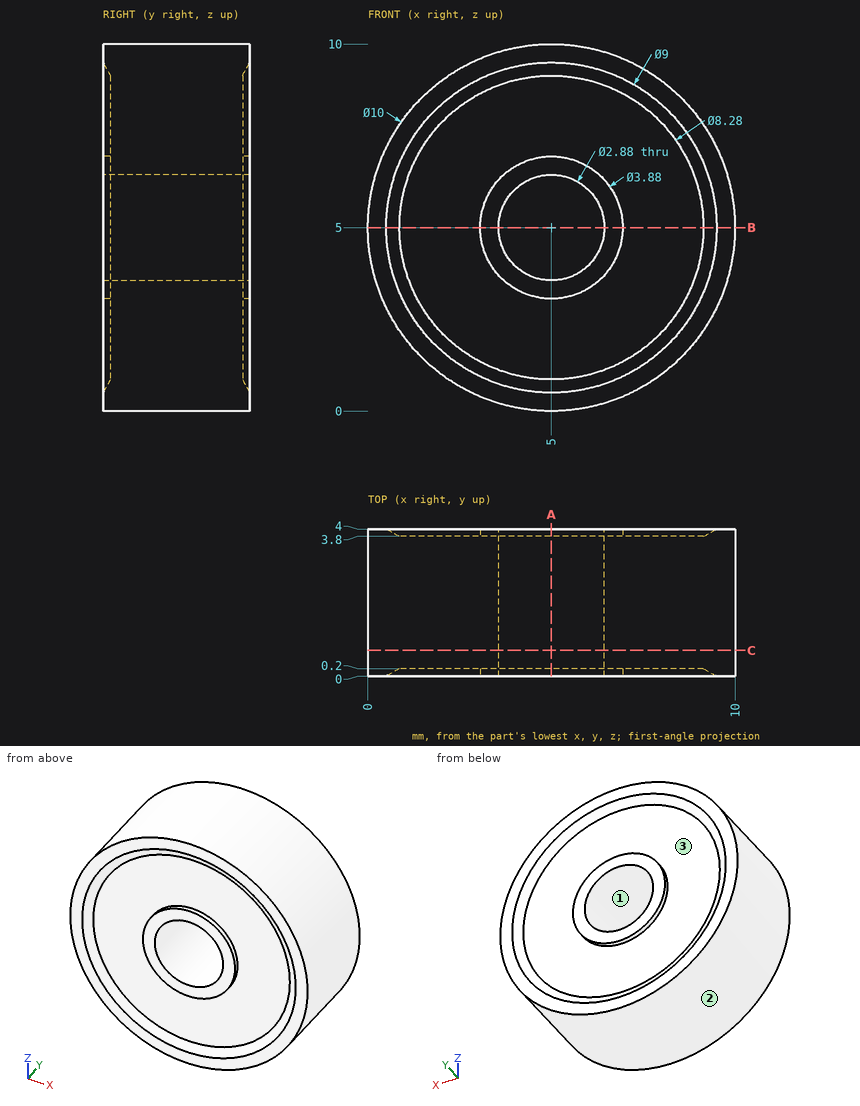
Study the drawing (mm; zero at the part's minimum x, y, z) and answer. Give positions to 0.01 mm unless a question says otherwise; leave off trailing zeros. Write each loop counter-clockwise with the first axis right and the second up, starting at its lowest first coordinate (ties: lowest second). Pieces come first, ordered by that corner, then holes.
Item 1: Flat-ended cylindrical pins translate along their axes: P1, Ø1.7, axis at x = 5, z = 5, coming from the +Y side; P2, Ø1, axis at y = 1.5, z = 7.5, coming from the +X side; P3, Ø1, axis at x = 1.5, z = 3.5, coming from the -Y side; P4, Ø1.5, axis at x = 2, z = 3.5, coming from the +Y side. Find the tip coordinate at first contact, or state that the pin passes through.
Item 2: Determine the mould class of the marked faces 1, 2 and 3 for opening direction Z: released by +Z, released by -Z, zero draft, split by the parting line, or undercut.
Item 3: Find the intervals of material crossed by line 1 along X through (y, z) = (2.65, 5); line 2 along Y through (x, z) = (9, 4.25); line 3 along Z through (x, y) = (5.5, 0.7), in increasing order.
Item 4: Section B-B, the plane z = 5 is taken. Write down the section's boundary in (x, y), plus the area to 3 significant figures.
Item 5: Section A-A, the plane x = 5 is taken. Write down the section's boundary in (y, z).
Item 6: Section C-C, the plane y = 0.7 is taken. Write down the section's boundary in (x, z).
Completed:
1. P1: passes through
1. P2: stops at x = 9.58
1. P3: stops at y = 0.11
1. P4: stops at y = 3.8
2. face 1: undercut
2. face 2: split by the parting line
2. face 3: undercut
3. line 1: x = 0 to 3.56, 6.44 to 10
3. line 2: y = 0.2 to 3.8
3. line 3: z = 0.03 to 3.65, 6.35 to 9.97
4. outline: (0, 0) - (0.5, 0) - (0.86, 0.2) - (3.06, 0.2) - (3.06, 0) - (3.56, 0) - (3.56, 4) - (3.06, 4) - (3.06, 3.8) - (0.86, 3.8) - (0.5, 4) - (0, 4) - close; (6.44, 0) - (6.94, 0) - (6.94, 0.2) - (9.14, 0.2) - (9.5, 0) - (10, 0) - (10, 4) - (9.5, 4) - (9.14, 3.8) - (6.94, 3.8) - (6.94, 4) - (6.44, 4) - close
4. area: 26.6 mm2
5. outline: (0, 0) - (4, 0) - (4, 0.5) - (3.8, 0.86) - (3.8, 3.06) - (4, 3.06) - (4, 3.56) - (0, 3.56) - (0, 3.06) - (0.2, 3.06) - (0.2, 0.86) - (0, 0.5) - close; (0, 6.44) - (4, 6.44) - (4, 6.94) - (3.8, 6.94) - (3.8, 9.14) - (4, 9.5) - (4, 10) - (0, 10) - (0, 9.5) - (0.2, 9.14) - (0.2, 6.94) - (0, 6.94) - close
6. outline: circle Ø10 at (5, 5); hole circle Ø2.88 at (5, 5)
